Work out the finished part from the listing and answer in its coordinate system (mm). A direction names the side the tool comes from. Round coordinates to 2 decimals unless told otherwise and drop trailing zeros. Order: outer loops, then holes, each group sorted by start corner. A loop starts at its lowest first (then second) coordinate and runs counter-clockwise, first axis right, second up. Notation, with made-up numbers: (-2.75, 56.25) -> (20.25, 56.25) arc R26 ccw to (20.25, 86.25) -> close; hole circle Ø1 at (-5.5, -26.75). An arc over 180 degrees is marked (long way). Use a Markdown table: item, result. Add a question column.
Item 1: A cutting plane is placed at A-A, the plane x = 7. Determine the outline of the cut face in (y, z), plus the area to 3 significant figures.
Item 2: A cutting plane is placed at C-C, the plane y = -5. Determine the outline of the cut face in (x, z), plus the area to 3 significant figures.
Item 3: Find the intervals of material crossed by L1, parallel to Y at x = -7, z = 24.75; L2, parallel to X at y = 0.75, z = -3.5; L3, parallel to X at y = -4.75, z = 17, in increasing order. Write a range as [from, to].
Item 4: For a pull along Z with two mould halves and no side action, classify faces 1 (the cylindrical face through (10.376, 2.986, -11.942)), 2 (the flat face through (0, 1, 8.5)), 3 (the cylindrical face through (-11.2, 2.99, 0.86)), 4 (the flat face through (-11, 4, -11)) as +Z half, -Z half, draft (parallel to the pull), parting line (faces both ways), or undercut.
Item 5: A cutting plane is placed at D-D, the plane z = 19. Determine the outline of the cut face in (x, y).
Item 6: A tool of negligible diameter and unlimited length cuts with its end or side. For faces 5 (the flat face through (0, -4, 12.5)), 6 (the cylindrical face through (-10.624, 2.986, -11.942)), 7 (the flat face through (-8.5, 1, -2)), 8 (the flat face through (12.5, -2, 16)), from which of +Z, -Z, +X, -X, +Y, -Y can it reach the whole face along a straight path? Write none if from no direction.
Item 7: A cutting plane is placed at B-B, the plane z = 1.5. Determine the outline of the cut face in (x, y).
Item 8: Flat-ended cylindrical pins translate along their axes: P1, Ø2, axis at x = -1.5, y = 1, coming from the -Z side; P2, Ø4, axis at y = -1, z = 9, coming from the +X side; P3, Ø3, axis at x = 2.5, z = 17.5, coming from the +Y side; P4, Ø3, axis at x = 9.5, z = 1, coming from the -Y side. Find the tip coordinate at first contact, or state that the pin passes through.
from build123d import *

# Parameters (mm, degrees)
BOSS_EXTRUDE1_DEPTH = 2
SKETCH2_R           = 0.95
BOSS_EXTRUDE2_DEPTH = 2
SKETCH3_W           = 25
SKETCH3_H           = 10
BOSS_EXTRUDE3_DEPTH = 15
SKETCH4_R           = 1.6
CUT_EXTRUDE1_DEPTH  = 20


with BuildPart() as part:
    # Sketch1 → Boss-Extrude1 (new body)
    with BuildSketch(Plane(origin=(0, 0, 0), x_dir=(1, 0, 0), z_dir=(0, 1, 0))):
        Polygon((-8.5, 12.5), (-8.5, -8.5), (8.5, -8.5), (8.5, 12.5), (12.5, 12.5), (12.5, -12.5), (-12.5, -12.5), (-12.5, 12.5), align=None)
    extrude(amount=BOSS_EXTRUDE1_DEPTH)

    # Sketch2 → Boss-Extrude2 (add)
    with BuildSketch(Plane(origin=(0, 2, 0), x_dir=(1, 0, 0), z_dir=(0, 1, 0))):
        with Locations((-10.5, 11)):
            Circle(SKETCH2_R)
        with Locations((-10.5, -1.5)):
            Circle(SKETCH2_R)
        with Locations((10.5, 11)):
            Circle(SKETCH2_R)
        with Locations((10.5, -1.5)):
            Circle(SKETCH2_R)
    extrude(amount=BOSS_EXTRUDE2_DEPTH)

    # Sketch3 → Boss-Extrude3 (add)
    with BuildSketch(Plane.XY.offset(12.5)):
        with Locations((0, -3)):
            Rectangle(SKETCH3_W, SKETCH3_H)
    extrude(amount=BOSS_EXTRUDE3_DEPTH)

    # Sketch4 → Cut-Extrude1 (cut)
    with BuildSketch(Plane.XY.offset(27.5)):
        with Locations((-7, -5)):
            Circle(SKETCH4_R)
        with Locations((7, -5)):
            Circle(SKETCH4_R)
    extrude(amount=-CUT_EXTRUDE1_DEPTH, mode=Mode.SUBTRACT)


solid = part.part
Reported:
| question | item | result |
|---|---|---|
| 1 | outline | (-8, 12.5) -> (-6.6, 12.5) -> (-6.6, 27.5) -> (-8, 27.5) -> close; (-3.4, 12.5) -> (0, 12.5) -> (0, 8.5) -> (2, 8.5) -> (2, 27.5) -> (-3.4, 27.5) -> close |
| 1 | area | 110 mm² |
| 2 | outline | (-12.5, 12.5) -> (-8.6, 12.5) -> (-8.6, 27.5) -> (-12.5, 27.5) -> close; (-5.4, 12.5) -> (5.4, 12.5) -> (5.4, 27.5) -> (-5.4, 27.5) -> close; (8.6, 12.5) -> (12.5, 12.5) -> (12.5, 27.5) -> (8.6, 27.5) -> close |
| 2 | area | 279 mm² |
| 3 | L1 | [-8, -6.6], [-3.4, 2] |
| 3 | L2 | [-12.5, -8.5], [8.5, 12.5] |
| 3 | L3 | [-12.5, -8.58], [-5.42, 5.42], [8.58, 12.5] |
| 4 | face 1 | undercut |
| 4 | face 2 | -Z half |
| 4 | face 3 | undercut |
| 4 | face 4 | draft |
| 5 | outline | (-12.5, -8) -> (12.5, -8) -> (12.5, 2) -> (-12.5, 2) -> close; hole circle Ø3.2 at (-7, -5); hole circle Ø3.2 at (7, -5) |
| 6 | face 5 | -Z, +X, -X, -Y |
| 6 | face 6 | +Y |
| 6 | face 7 | -Z, +Y, -Y |
| 6 | face 8 | +Z, -Z, +X, +Y, -Y |
| 7 | outline | (-12.5, 0) -> (-8.5, 0) -> (-8.5, 2) -> (-9.55, 2) -> (-9.55, 4) -> (-11.45, 4) -> (-11.45, 2) -> (-12.5, 2) -> close; (8.5, 0) -> (12.5, 0) -> (12.5, 2) -> (11.45, 2) -> (11.45, 4) -> (9.55, 4) -> (9.55, 2) -> (8.5, 2) -> close |
| 8 | P1 | z = 8.5 |
| 8 | P2 | x = 12.5 |
| 8 | P3 | y = 2 |
| 8 | P4 | y = 0 |
